Could you check a few things on this model? Use its own coordinates, in mm. Face numbers are marked on the shaded views. A direction names the side the tool comes from. Round coordinates to 2 decimals unless told otherwise and drop trailing zeros. Write each loop counter-clockwise with the first axis right and the second up, starting at its lowest first coordinate (ties: lowest second). Pieces come first, ordered by that corner, then holes. Notation, with made-up numbers: (25, -11.75) -> (36, -11.75) arc R8 ccw to (36, -4.75) -> close; hole circle Ø7 at (17, 51.25). An arc over 180 degrees is marked (long way). Answer in a Markdown table with one row per item. Add a question column.
```python
from build123d import *

# Parameters (mm, degrees)
SKETCH001_W     = 45
SKETCH001_H     = 23
PAD001_DEPTH    = 17
SKETCH002_W     = 41
SKETCH002_H     = 13
POCKET_DEPTH    = 21
SKETCH003_R     = 19.5
POCKET001_DEPTH = 17.001
CHAMFER_SIZE    = 1.5


with BuildPart() as part:
    # Sketch001 → Pad001 (new body)
    with BuildSketch(Plane.XY):
        with Locations((0, -11.5)):
            Rectangle(SKETCH001_W, SKETCH001_H)
    extrude(amount=PAD001_DEPTH)

    # Sketch002 (on Face1 of Pad001) → Pocket (cut)
    with BuildSketch(Plane(origin=(0, 0, 0), x_dir=(-1, 0, 0), z_dir=(0, 1, 0))):
        with Locations((0, 8.5)):
            Rectangle(SKETCH002_W, SKETCH002_H)
    extrude(amount=-POCKET_DEPTH, mode=Mode.SUBTRACT)

    # Sketch003 (on Face4 of Pocket) → Pocket001 (cut, through all)
    with BuildSketch(Plane.XY.offset(17)):
        Circle(SKETCH003_R)
    extrude(amount=-POCKET001_DEPTH, mode=Mode.SUBTRACT)

    # Chamfer
    chamfer_edges = [part.edges().sort_by_distance(p)[0] for p in [
        (-22.5, -23, 8.5),
        (22.5, -23, 8.5),
    ]]
    chamfer(chamfer_edges, length=CHAMFER_SIZE)


solid = part.part
```
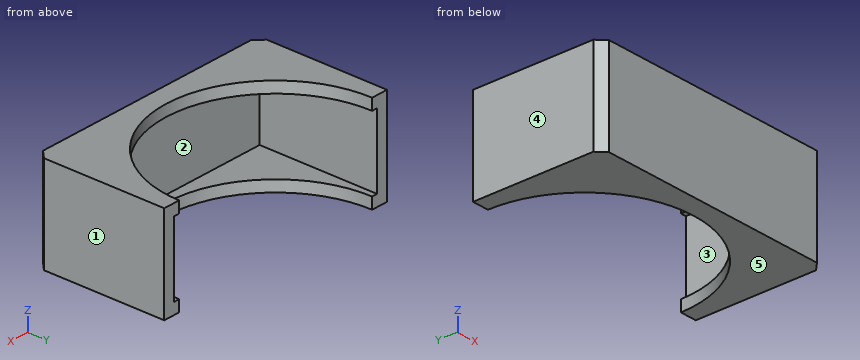
(1) I need wall thicknesses on L1, parallel to Z at x = -14, y = -20; L2, parallel to X at y = -5, z = 9.5; L3, parallel to Y at x = 4.5, z = 12.75. Which ranges of each line are inside material? Lowest first, please.
(2) Suppose I cut it at D-D, the plane z = 3.75. Please give me the cut outline in (x, y), then the cut area to 3 significant figures.
(3) For P1, Ø1.5, axis at x = -8, z = 5.5, coming from the +Y side, with a flat end and sliding along its axis, tell me the tip position at first contact or that it passes through.
(4) Suppose I cut it at A-A, the plane y = -20.25. Please give me the cut outline in (x, z).
(5) On a 3-axis mill with a long thin cutter (end or side, diameter ignored), from which of +Z, -Z, +X, -X, +Y, -Y can I reach the whole of each face in a straight line? I mean the marked faces 1 and 2. Say none if no direction works.
(6) Suppose I cut it at C-C, the plane y = -12.5. Please give me the cut outline in (x, z).
(7) If we mould it in two halves opening along X, with no side actions, what happens to the marked faces 3, 4 and 5? For each: pulls with the +X half, pulls with the -X half, needs draft (parallel to the pull), parting line crosses it, or undercut.
(8) Suppose I cut it at B-B, the plane x = 0. Please give me the cut outline in (y, z), then the cut area to 3 significant figures.
Response:
| question | item | result |
|---|---|---|
| 1 | L1 | 0 to 2, 15 to 17 |
| 1 | L2 | -22.5 to -20.5, 20.5 to 22.5 |
| 1 | L3 | -23 to -21 |
| 2 | outline | (-22.5, -21.5) -> (-21, -23) -> (21, -23) -> (22.5, -21.5) -> (22.5, 0) -> (20.5, 0) -> (20.5, -21) -> (-20.5, -21) -> (-20.5, 0) -> (-22.5, 0) -> close |
| 2 | area | 172 mm² |
| 3 | P1 | y = -21 |
| 4 | outline | (-22.5, 0) -> (22.5, 0) -> (22.5, 17) -> (-22.5, 17) -> close; hole (-20.5, 2) -> (20.5, 2) -> (20.5, 15) -> (-20.5, 15) -> close |
| 5 | face 1 | +Z, -Z, +X, +Y, -Y |
| 5 | face 2 | +Y |
| 6 | outline | (-22.5, 0) -> (-14.97, 0) -> (-14.97, 2) -> (-20.5, 2) -> (-20.5, 15) -> (-14.97, 15) -> (-14.97, 17) -> (-22.5, 17) -> close; (14.97, 0) -> (22.5, 0) -> (22.5, 17) -> (14.97, 17) -> (14.97, 15) -> (20.5, 15) -> (20.5, 2) -> (14.97, 2) -> close |
| 7 | face 3 | undercut |
| 7 | face 4 | pulls with the -X half |
| 7 | face 5 | needs draft |
| 8 | outline | (-23, 0) -> (-19.5, 0) -> (-19.5, 2) -> (-21, 2) -> (-21, 15) -> (-19.5, 15) -> (-19.5, 17) -> (-23, 17) -> close |
| 8 | area | 40.0 mm² |
